Autodesk Inventor part; units mm, degrees
ref_plane "YZ Plane" through (0, 0, 0) normal (1, 0, 0) x (0, 1, 0)
ref_plane "XZ Plane" through (0, 0, 0) normal (0, 1, 0) x (-1, 0, 0)
ref_plane "XY Plane" through (0, 0, 0) normal (0, 0, 1) x (1, 0, 0)
sketch "Boceto1" plane through (0, 0, 0) normal (1, 0, 0) x (0, 1, 0)
  line L0 (10, -25) -> (10, -70)
  line L1 (10, -70) -> (38, -70)
  line L2 (38, -70) -> (38, -60)
  line L3 (38, -60) -> (18, -60)
  line L4 (18, -60) -> (18, 0)
  line L5 (18, 0) -> (13, 0)
  line L6 (-7.6, 0) -> (45.6, 0) construction
  line L7 (0, -84) -> (0, 14)
  line L8 (13, 0) -> (13, -25)
  line L9 (13, -25) -> (10, -25)
  point P0 (0, 0)
  dimension "d6" = 20
  dimension "d8" = 36
  dimension "d9" = 10
  dimension "d10" = 76
  dimension "d11" = 26
  dimension "d12" = 25
  dimension "d35" = 70
revolve "Revolución1" add sketch "Boceto1" angle 360 about axis through (0, 0, -10) along (0, 0, 1)
sketch "Boceto2" plane through (0, 0, 0) normal (0, 0, 1) x (1, 0, 0)
  line L0 (-53.2, 0) -> (53.2, 0) construction
  line L1 (0, -70) -> (0, 70) construction
  arc A0 (11.2759, 42.1053) -> (-11.2759, 42.1053) centre (0, 38) ccw
  line L2 (-11.2759, 42.1053) -> (-23.4915, 8.5526)
  line L3 (11.2759, 42.1053) -> (23.4915, 8.5526)
  arc A1 (-23.4915, 8.5526) -> (-25, 0) centre (0, 0) ccw
  arc A2 (25, 0) -> (23.4915, 8.5526) centre (0, 0) ccw
  circle A3 centre (0, 38) radius 5
  arc A4 (-11.2759, -42.1053) -> (11.2759, -42.1053) centre (0, -38) ccw
  line L4 (-11.2759, -42.1053) -> (-23.4915, -8.5526)
  line L5 (11.2759, -42.1053) -> (23.4915, -8.5526)
  arc A5 (-25, 0) -> (-23.4915, -8.5526) centre (0, 0) ccw
  arc A6 (23.4915, -8.5526) -> (25, 0) centre (0, 0) ccw
  circle A7 centre (0, -38) radius 5
  circle A8 centre (0, 0) radius 13
  dimension "d14" = 12
  dimension "d15" = 25
  dimension "d16" = 38
  dimension "d17" = 10
extrude "Extrusión1" add sketch "Boceto2" against normal blind 12
sketch "Boceto3" plane through (0, 0, -70) normal (0, 0, -1) x (-1, 0, 0)
  circle A0 centre (0, 0) radius 29 construction
  point P0 (0, 29)
  dimension "d20" = 58
hole "Agujero1" at (0, 29, -70) direction (0, 0, 1) diameter 8 depth 10
pattern_circular "Patrón circular1" count 6 over 360 about axis through (0, 0, -10) along (0, 0, 1) of "Agujero1"
chamfer "Chaflán1" distance 3 angle 45 1 edges at (0, -13, 0) measured on face at (11.9516, -17.6559, 0)
fillet "Empalme1" radius 2 2 edges at (0, -18, -60) (0, -38, -60)
properties part number "Lab6A01209499P1" material "Hierro, fundido"
Read the model definition and answer for the solid it produces. Units are mm, in the model's axes. A direction names the side the tool comes from. Round coordinates to 2 decimals unless told otherwise and drop trailing zeros. Order: outer loops, then holes, each group sorted by start corner. A loop starts at its lowest first (then second) coordinate and runs counter-clockwise, first axis right, second up.
1) For faces 4 (the face through (-17.3, 25.56, -5.92)), 5 (the face through (24.61, -4.4, -5.92)), 6 (the face through (16.3, -0.7, 0)), 7 (the face through (2.4, 25.8, -64.9)), 8 (the face through (3, -34, -6)), determine the directions among +Z, -Z, +X, -X, +Y, -Y from which every point of the face is accessible in a straight line to the end or side of a thin tool.
2) The part is cut by section A-A on z = -9.5. Write down the section's boundary in (x, y).
3) Flat-ended cylindrical pins translate along their axes: pin 1 (1.5 mm diameter, centred on y = 9, z = -7.5, fed in from +X); pin 2 (4 mm diameter, centred on y = -1.5, z = -57.5, fed in from -X); pin 3 (1 mm diameter, centred on y = -10, z = -56.5, fed in from -X). Find the tip coordinate at first contact, or state that the pin passes through.
4) The part is cut by section B-B on x = 0. Give the number of separate pieces and of enclosed holes in the cut face, plus the area to 3 significant figures.
5) Straight lines are drawn through the part: L1, parallel to Z at x = -6, y = -32.5; L2, parallel to X at y = -14, z = -67; L3, parallel to X at y = 0, z = -9. For each, find the intervals that lie inside material, in ascending order.
6) The mould has two halves that part along Y. Classify faces 1 (the face through (17.3, -25.56, -5.92)), 2 (the face through (16, -10, -12)), 3 (the face through (28.66, -12.65, -64.93)): released by +Y, released by -Y, zero draft, split by the parting line, or undercut.
7) The part is cut by section D-D on z = -63.5. Write down the section's boundary in (x, y), plus the area to 3 significant figures.
Resolved:
1. face 4: +Z, -X, +Y
1. face 5: +Z, +X, -Y
1. face 6: +Z, +X, -X, +Y, -Y
1. face 7: -Z
1. face 8: +Z
2. outline: (-25, 0) arc R25 ccw to (-23.49, -8.55) - (-11.28, -42.11) arc R12 ccw to (11.28, -42.11) - (23.49, -8.55) arc R25 ccw to (25, 0) arc R25 ccw to (23.49, 8.55) - (11.28, 42.11) arc R12 ccw to (-11.28, 42.11) - (-23.49, 8.55) arc R25 ccw to start; hole circle Ø26 at (0, 0); hole circle Ø10 at (0, -38); hole circle Ø10 at (0, 38)
3. pin 1: stops at x = 23.6
3. pin 2: stops at x = -18.62
3. pin 3: stops at x = -15.29
4. separate pieces: 6
4. enclosed holes: 0
4. area: 1,730 mm2
5. L1: z = -70 to -60, -12 to 0
5. L2: x = -35.33 to -29.08, -21.15 to 21.15, 29.08 to 35.33
5. L3: x = -25 to -13, 13 to 25
6. face 1: released by -Y
6. face 2: zero draft
6. face 3: undercut
7. outline: circle Ø76 at (0, 0); hole circle Ø8 at (-25.11, -14.5); hole circle Ø8 at (-25.11, 14.5); hole circle Ø20 at (0, 0); hole circle Ø8 at (0, -29); hole circle Ø8 at (0, 29); hole circle Ø8 at (25.11, -14.5); hole circle Ø8 at (25.11, 14.5)
7. area: 3,920 mm2
